Check sheet for the modelled part. Datum: model origin and axes. Units: mm. A direction names the side the tool comes from. Round coordinates to 2 decimals unless told otherwise and drop trailing zeros. Loops run counter-clockwise (first coordinate to the right, second up) from the corner with the lowest first, then second, coordinate; pieces in that order, holes last. Notation, with made-up numbers: M 57.25,-39.5 L 64.25,-39.5 A12 ccw 64.25,-21.5 Z; hole C -9,13.5 d1. An arc over 180 degrees is marked long. One line per question, with ' | ' between items. Start each with the question number.
(1) Section check D-D (y = 23.5). Record the boundary of the cut face in (x, z), and give its area (3 significant figures).
(2) Go/stop test with flat-tipped pins: P1, Ø1.5, axis at y = 32, z = 47, coming from the +X side; P2, Ø1, axis at x = -6.5, z = 68, coming from the -Y side; P3, Ø2, axis at x = -4, z = 45.5, coming from the +Y side; P4, Ø10, axis at x = 5, y = -19.5, coming from the -Z side. Record where each tip stops, or that it passes through.
(3) Tool access check on faces 1 (the face through (6.9, 41.181, 74.336)), 2 (the face through (-1, 1, 0)). Record the directions out of +Z, -Z, +X, -X, +Y, -Y that give a thin tool (end or side, any length) a straight path to the whole face; none if there is none.
(4) Thickness scan on probe 1 along Y at (x, z) = (0, 93); probe 2 along Z at (x, y) = (36, 13); probe 3 along Y at (x, z) = (12, 87). Record the ranges inside material, lowest first. Write a range as [from, to].
(5) Section check C-C (z = 114.5). Record the boundary of the cut face in (x, y).
(6) Draft check along Y on faces 3 (the face through (-5.66, 43.13, 61.13)), 4 (the face through (-8.78, -39.537, 63.667)), 5 (the face through (29, -29, 124)), 6 (the face through (-1, 1, 5)). Enter one of: +Y half, -Y half, draft (parallel to the pull), parting line (faces both ways), or undercut.
(7) Section check A-A (y = 0). Record the boundary of the cut face in (x, z).
(8) Section check B-B (x = -2). Record the boundary of the cut face in (y, z).
```python
from build123d import *

# Parameters (mm, degrees)
F0_R     = 43.5
F0_R_2   = 40.5
F1_DEPTH = 124
F2_DEPTH = 5
F4_DEPTH = 43.501


with BuildPart() as f1:
    # F0 (on Top) → F1 (new body)
    with BuildSketch(Plane.XY):
        Circle(F0_R)
        Circle(F0_R_2, mode=Mode.SUBTRACT)
    extrude(amount=F1_DEPTH)

    # F0 (on Top) → F2 (join)
    with BuildSketch(Plane.XY):
        Circle(F0_R_2)
    extrude(amount=F2_DEPTH)

    # F3 (on Front) → F4 (cut, through all)
    with BuildSketch(Plane.XZ):
        with BuildLine():
            Line((-11.173021, 68.756767), (0, 55.116978))
            Line((0, 55.116978), (11.180688, 68.750483))
            ThreePointArc((11.180688, 68.750483), (6.798893, 74.367971), (0, 72.239272))
            ThreePointArc((0, 72.239272), (-6.790198, 74.359844), (-11.173021, 68.756767))
        make_face()
    extrude(amount=-F4_DEPTH, mode=Mode.SUBTRACT)


solid = f1.part
```
The answers:
1) outline: M -36.61,0 L 36.61,0 L 36.61,124 L 32.98,124 L 32.98,5 L -32.98,5 L -32.98,124 L -36.61,124 Z | area: 1,230 mm²
2) P1: x = 30.26 | P2: y = -43.08 | P3: y = 43.4 | P4: z = 0
3) face 1: +Y | face 2: -Z, +X, -X, +Y, -Y
4) probe 1: [-43.5, -40.5], [40.5, 43.5] | probe 2: [0, 5] | probe 3: [-41.81, -38.68], [38.68, 41.81]
5) outline: C 0,0 d87; hole C 0,0 d81
6) face 3: parting line | face 4: undercut | face 5: draft | face 6: undercut
7) outline: M -43.5,0 L 43.5,0 L 43.5,124 L 40.5,124 L 40.5,5 L -40.5,5 L -40.5,124 L -43.5,124 Z
8) outline: M -43.45,0 L 43.45,0 L 43.45,57.56 L 40.45,57.56 L 40.45,5 L -40.45,5 L -40.45,124 L -43.45,124 Z; M 40.45,73.92 L 43.45,73.92 L 43.45,124 L 40.45,124 Z
